Geometry: final body of the model. Coordinates: model frame, mm. A direction names the side the tool comes from. Give positions to 0.01 mm unless a question says otherwise; leave off trailing zeros. Write each loop counter-clockwise with the first axis right and the second up, starting at its lowest first coordinate (ties: lowest second). Pieces come first, ordered by that corner, then holes. Notation, with made-up numbers: (-22, -28) -> (27, -28) arc R34 cw to (27, 5) -> close; hole circle Ø6 at (8.25, 64.25). An arc over 180 degrees is marked (long way). Answer as a JSON object with one key per item and string values.
from build123d import *

# Parameters (mm, degrees)
SKETCH1_W           = 39
SKETCH1_H           = 22
SKETCH1_R           = 2
BOSS_EXTRUDE1_DEPTH = 5
SKETCH4_R           = 4
BOSS_EXTRUDE2_DEPTH = 6
BOSS_EXTRUDE3_DEPTH = 5


with BuildPart() as part:
    # Sketch1 → Boss-Extrude1 (new body)
    with BuildSketch(Plane(origin=(0, 0, 0), x_dir=(1, 0, 0), z_dir=(0, 1, 0))):
        with Locations((10.5, 1)):
            Rectangle(SKETCH1_W, SKETCH1_H)
        with Locations(Location((0, 0, 0), (0, 0, 270))):
            Circle(SKETCH1_R, mode=Mode.SUBTRACT)
        with Locations(Location((17, 0, 0), (0, 0, 270))):
            Circle(SKETCH1_R, mode=Mode.SUBTRACT)
    extrude(amount=BOSS_EXTRUDE1_DEPTH)

    # Sketch4 → Boss-Extrude2 (add)
    with BuildSketch(Plane(origin=(0, 0, -12), x_dir=(-1, 0, 0), z_dir=(0, 0, -1))):
        Polygon((-30, 5), (9, 5), (9, 15), (9, 95), (-30, 95), (-30, 15), align=None)
        with Locations((-16, 87)):
            Circle(SKETCH4_R, mode=Mode.SUBTRACT)
    extrude(amount=-BOSS_EXTRUDE2_DEPTH)

    # Sketch5 → Boss-Extrude3 (add)
    with BuildSketch(Plane(origin=(30, 0, 0), x_dir=(0, 0, -1), z_dir=(1, 0, 0))):
        Polygon((-10, 5), (6, 5), (6, 20), align=None)
    extrude(amount=-BOSS_EXTRUDE3_DEPTH)


solid = part.part
Q1. First-contact query: P1, Ø5, axis at x = 8, z = -0.5, coming from the +Y side; P2, Ø19.5, axis at x = 16.5, y = 63, coming from the +Z side; P3, Ø3, axis at x = 0, z = 0, coming from the -Y side; P4, Ø10, axis at y = 34, z = -2, coming from the +X side. Flat tips, straight axial feed; report the tip coordinate or a pass-through.
Values:
{"P1": "y = 5", "P2": "z = -6", "P3": "through", "P4": "x = 30"}
Q2. Cut plane A-A (x = 0). Return the cut outline in (y, z).
Values:
{"outline": "(0, -12) -> (95, -12) -> (95, -6) -> (5, -6) -> (5, -2) -> (0, -2) -> close; (0, 2) -> (5, 2) -> (5, 10) -> (0, 10) -> close"}
Q3. Cut plane C-C (x = 17). Return the cut outline in (y, z), and give its area (3 significant figures).
Values:
{"outline": "(0, -12) -> (83.13, -12) -> (83.13, -6) -> (5, -6) -> (5, -2) -> (0, -2) -> close; (0, 2) -> (5, 2) -> (5, 10) -> (0, 10) -> close; (90.87, -12) -> (95, -12) -> (95, -6) -> (90.87, -6) -> close", "area": "584 mm²"}
Q4. Set-up query: faces 5 (the flat face through (8, 5, 2)), 6 (the cylindrical face through (16.867, 83.095, -9.042)). Return all of +Z, -Z, +X, -X, +Y, -Y with unobstructed straight access to the full face (end or side cutting, diameter ignored); none if empty.
Values:
{"face 5": "+Z, -X, +Y", "face 6": "+Z, -Z"}
Q5. Cut plane B-B (y = 87). Return the cut outline in (x, z), and give its area (3 significant figures).
Values:
{"outline": "(-9, -12) -> (12, -12) -> (12, -6) -> (-9, -6) -> close; (20, -12) -> (30, -12) -> (30, -6) -> (20, -6) -> close", "area": "186 mm²"}
Q6. Mould query, pull axis X, two halves, no side actions, for faces 1 (the cylindrical face through (19, 2, 0)), 2 (the cylindrical face through (-2, 2, 0)), 3 (the flat face through (11, 48, -12)), 4 (the flat face through (30, 37, -7)). Classes: pulls with the +X half, pulls with the -X half, needs draft (parallel to the pull), parting line crosses it, or undercut.
Values:
{"face 1": "undercut", "face 2": "undercut", "face 3": "needs draft", "face 4": "pulls with the +X half"}
Q7. Cut plane D-D (z = 0). Return the cut outline in (x, y) (3 decimals).
Values:
{"outline": "(-9, 0) -> (-2, 0) -> (-2, 5) -> (-9, 5) -> close; (2, 0) -> (15, 0) -> (15, 5) -> (2, 5) -> close; (19, 0) -> (30, 0) -> (30, 14.375) -> (25, 14.375) -> (25, 5) -> (19, 5) -> close"}
Q8. Material intervals for L1, parallel to X at y = 1.35, z = 0; L2, parallel to Y at x = 16, z = -8.75; L3, parallel to Z at x = -3, y = 80, sorted ascending. Write a range as from..to.
Values:
{"L1": "-9..-2, 2..15, 19..30", "L2": "0..83, 91..95", "L3": "-12..-6"}
